from build123d import *

# Parameters (mm, degrees)
SKETCH1_W                   = 36
SKETCH1_H                   = 38
BOSS_EXTRUDE2_DEPTH         = 53
SKETCH3_W                   = 30
SKETCH3_H                   = 35
CUT_EXTRUDE1_DEPTH          = 51
SKETCH4_W                   = 3
SKETCH4_H                   = 30
BOSS_EXTRUDE3_DEPTH         = 33
SKETCH5_W                   = 53
SKETCH5_H                   = 8
CUT_EXTRUDE2_DEPTH          = 52
SKETCH6_W                   = 53
SKETCH6_H                   = 7
BOSS_EXTRUDE4_DEPTH         = 3
CUT_EXTRUDE4_DEPTH          = 79.797208072
CUT_EXTRUDE4_DEPTH_BACK     = 79.797208072
SKETCH8_W                   = 11.5
SKETCH8_H                   = 3
M3_TAPPED_HOLE1_D           = 2.5
M3_TAPPED_HOLE1_DEPTH       = 3
M3_TAPPED_HOLE1_CSINK_D     = 3.05
M3_TAPPED_HOLE1_CSINK_ANGLE = 179
LPATTERN1_COUNT             = 2
LPATTERN1_PITCH             = 24
LPATTERN1_COUNT_DIR2        = 2
LPATTERN1_PITCH_DIR2        = 12
M3_TAPPED_HOLE2_D           = 2.5
M3_TAPPED_HOLE2_DEPTH       = 2
M3_TAPPED_HOLE2_CSINK_D     = 3.05
M3_TAPPED_HOLE2_CSINK_ANGLE = 179
LPATTERN2_COUNT             = 2
LPATTERN2_PITCH             = 16
LPATTERN2_COUNT_DIR2        = 2
LPATTERN2_PITCH_DIR2        = 12
M3_TAPPED_HOLE3_D           = 2.5
M3_TAPPED_HOLE3_CSINK_D     = 3.05
M3_TAPPED_HOLE3_CSINK_ANGLE = 179
LPATTERN3_COUNT             = 2
LPATTERN3_PITCH             = 16
M3_TAPPED_HOLE4_D           = 2.5
M3_TAPPED_HOLE4_CSINK_D     = 3.05
M3_TAPPED_HOLE4_CSINK_ANGLE = 179
LPATTERN4_COUNT             = 2
LPATTERN4_PITCH             = 24
LPATTERN4_COUNT_DIR2        = 2
LPATTERN4_PITCH_DIR2        = 12
SKETCH45_R                  = 1.833333333
CUT_EXTRUDE5_DEPTH          = 74.396185187
LPATTERN5_COUNT             = 2
LPATTERN5_PITCH             = 35
LPATTERN5_COUNT_DIR2        = 2
LPATTERN5_PITCH_DIR2        = 43
CUT_EXTRUDE6_DEPTH          = 75.551995278
CUT_EXTRUDE6_DEPTH_BACK     = 75.551995278
SKETCH46_W                  = 11.5
SKETCH46_H                  = 3.2
CUT_EXTRUDE7_DEPTH          = 74.396185187
CUT_EXTRUDE7_DEPTH_BACK     = 74.396185187
SKETCH47_W                  = 53
SKETCH47_H                  = 7
BOSS_EXTRUDE5_START         = -30
SKETCH49_W                  = 10
SKETCH49_H                  = 36
BOSS_EXTRUDE5_DEPTH         = 3
CUT_EXTRUDE8_DEPTH          = 78.420927403
CUT_EXTRUDE8_DEPTH_BACK     = 78.420927403
SKETCH50_R                  = 1.835


with BuildPart() as part:
    # Sketch1 → Boss-Extrude2 (new body)
    with BuildSketch(Plane(origin=(0, 0, 0), x_dir=(0, 0, -1), z_dir=(1, 0, 0))):
        with Locations((18, 19)):
            Rectangle(SKETCH1_W, SKETCH1_H)
    extrude(amount=BOSS_EXTRUDE2_DEPTH)

    # Sketch3 → Cut-Extrude1 (cut)
    with BuildSketch(Plane(origin=(53, 0, 0), x_dir=(0, 0, -1), z_dir=(1, 0, 0))):
        with Locations((18, 17.5)):
            Rectangle(SKETCH3_W, SKETCH3_H)
    extrude(amount=-CUT_EXTRUDE1_DEPTH, mode=Mode.SUBTRACT)

    # Sketch4 → Boss-Extrude3 (add)
    with BuildSketch(Plane.XY):
        with Locations((51.5, 15)):
            Rectangle(SKETCH4_W, SKETCH4_H)
    extrude(amount=-BOSS_EXTRUDE3_DEPTH)

    # Sketch5 → Cut-Extrude2 (cut)
    with BuildSketch(Plane.XY):
        with Locations((26.5, 34)):
            Rectangle(SKETCH5_W, SKETCH5_H)
    extrude(amount=-CUT_EXTRUDE2_DEPTH, mode=Mode.SUBTRACT)

    # Sketch6 → Boss-Extrude4 (add)
    with BuildSketch(Plane(origin=(0, 0, 0), x_dir=(-1, 0, 0), z_dir=(0, -1, 0))):
        with Locations((-26.5, -3.5)):
            Rectangle(SKETCH6_W, SKETCH6_H)
        with Locations((-26.5, 39.5)):
            Rectangle(SKETCH6_W, SKETCH6_H)
    extrude(amount=-BOSS_EXTRUDE4_DEPTH)

    # Sketch8 → Cut-Extrude4 (cut, two sides: drawn at the far end of the back side and taken through both)
    with BuildSketch(Plane(origin=(0, 0, -43), x_dir=(-1, 0, 0), z_dir=(0, 0, -1)).offset(-CUT_EXTRUDE4_DEPTH_BACK)):
        with Locations((-23.75, 1.5)):
            Rectangle(SKETCH8_W, SKETCH8_H)
    extrude(amount=CUT_EXTRUDE4_DEPTH + CUT_EXTRUDE4_DEPTH_BACK, mode=Mode.SUBTRACT)

    # M3 Tapped Hole1
    with Locations(Plane.XY):
        with Locations((10, 23)):
            m3_tapped_hole1 = CounterSinkHole(M3_TAPPED_HOLE1_D / 2, M3_TAPPED_HOLE1_CSINK_D / 2, depth=M3_TAPPED_HOLE1_DEPTH, counter_sink_angle=M3_TAPPED_HOLE1_CSINK_ANGLE)

    # LPattern1: M3 Tapped Hole1 2 × 2
    with Locations(*[(i * LPATTERN1_PITCH, -j * LPATTERN1_PITCH_DIR2, 0) for i in range(LPATTERN1_COUNT) for j in range(LPATTERN1_COUNT_DIR2) if (i, j) != (0, 0)]):
        add(m3_tapped_hole1, mode=Mode.SUBTRACT)

    # M3 Tapped Hole2
    with Locations(Plane.ZY):
        with Locations((-26, 23)):
            m3_tapped_hole2 = CounterSinkHole(M3_TAPPED_HOLE2_D / 2, M3_TAPPED_HOLE2_CSINK_D / 2, depth=M3_TAPPED_HOLE2_DEPTH, counter_sink_angle=M3_TAPPED_HOLE2_CSINK_ANGLE)

    # LPattern2: M3 Tapped Hole2 2 × 2
    with Locations(*[(0, -j * LPATTERN2_PITCH_DIR2, i * LPATTERN2_PITCH) for i in range(LPATTERN2_COUNT) for j in range(LPATTERN2_COUNT_DIR2) if (i, j) != (0, 0)]):
        add(m3_tapped_hole2, mode=Mode.SUBTRACT)

    # M3 Tapped Hole3 (through all)
    with Locations(Plane(origin=(53, 0, 0), x_dir=(0, 0, -1), z_dir=(1, 0, 0))):
        with Locations((26, 23)):
            m3_tapped_hole3 = CounterSinkHole(M3_TAPPED_HOLE3_D / 2, M3_TAPPED_HOLE3_CSINK_D / 2, counter_sink_angle=M3_TAPPED_HOLE3_CSINK_ANGLE)

    # LPattern3: M3 Tapped Hole3 ×2
    with Locations(*[(0, 0, i * LPATTERN3_PITCH) for i in range(1, LPATTERN3_COUNT)]):
        add(m3_tapped_hole3, mode=Mode.SUBTRACT)

    # M3 Tapped Hole4 (through all)
    with Locations(Plane(origin=(0, 0, -36), x_dir=(-1, 0, 0), z_dir=(0, 0, -1))):
        with Locations((-10, 23)):
            m3_tapped_hole4 = CounterSinkHole(M3_TAPPED_HOLE4_D / 2, M3_TAPPED_HOLE4_CSINK_D / 2, counter_sink_angle=M3_TAPPED_HOLE4_CSINK_ANGLE)

    # LPattern4: M3 Tapped Hole4 2 × 2
    with Locations(*[(i * LPATTERN4_PITCH, -j * LPATTERN4_PITCH_DIR2, 0) for i in range(LPATTERN4_COUNT) for j in range(LPATTERN4_COUNT_DIR2) if (i, j) != (0, 0)]):
        add(m3_tapped_hole4, mode=Mode.SUBTRACT)

    # Sketch45 → Cut-Extrude5 (cut, symmetric)
    with BuildSketch(Plane(origin=(0, 3, 0), x_dir=(1, 0, 0), z_dir=(0, 1, 0))):
        with Locations(Location((8, 39.5, 0), (0, 0, 270))):
            Circle(SKETCH45_R)
    cut_extrude5 = extrude(amount=CUT_EXTRUDE5_DEPTH, both=True, mode=Mode.SUBTRACT)

    # LPattern5: Cut-Extrude5 2 × 2
    with Locations(*[(i * LPATTERN5_PITCH, 0, j * LPATTERN5_PITCH_DIR2) for i in range(LPATTERN5_COUNT) for j in range(LPATTERN5_COUNT_DIR2) if (i, j) != (0, 0)]):
        add(cut_extrude5, mode=Mode.SUBTRACT)

    # Sketch46 → Cut-Extrude6 (cut, two sides: drawn at the far end of the back side and taken through both)
    with BuildSketch(Plane(origin=(0, 0, -36), x_dir=(-1, 0, 0), z_dir=(0, 0, -1)).offset(-CUT_EXTRUDE6_DEPTH_BACK)):
        with Locations((-23.75, 4.6)):
            Rectangle(SKETCH46_W, SKETCH46_H)
    extrude(amount=CUT_EXTRUDE6_DEPTH + CUT_EXTRUDE6_DEPTH_BACK, mode=Mode.SUBTRACT)

    # Sketch47 → Cut-Extrude7 (cut, two sides: drawn at the far end of the back side and taken through both)
    with BuildSketch(Plane(origin=(0, 3, 0), x_dir=(1, 0, 0), z_dir=(0, 1, 0)).offset(-CUT_EXTRUDE7_DEPTH_BACK)):
        with Locations((26.5, 39.5)):
            Rectangle(SKETCH47_W, SKETCH47_H)
        with Locations((26.5, -3.5)):
            Rectangle(SKETCH47_W, SKETCH47_H)
    extrude(amount=CUT_EXTRUDE7_DEPTH + CUT_EXTRUDE7_DEPTH_BACK, mode=Mode.SUBTRACT)

    # Sketch49 → Boss-Extrude5 (add)
    with BuildSketch(Plane(origin=(0, 30, 0), x_dir=(1, 0, 0), z_dir=(0, 1, 0)).offset(BOSS_EXTRUDE5_START)):
        with Locations((-5, 18)):
            Rectangle(SKETCH49_W, SKETCH49_H)
        with Locations((58, 18)):
            Rectangle(SKETCH49_W, SKETCH49_H)
    extrude(amount=BOSS_EXTRUDE5_DEPTH)

    # Sketch50 → Cut-Extrude8 (cut, two sides: drawn at the far end of the back side and taken through both)
    with BuildSketch(Plane(origin=(0, 3, 0), x_dir=(1, 0, 0), z_dir=(0, 1, 0)).offset(-CUT_EXTRUDE8_DEPTH_BACK)):
        with Locations(Location((-5, 28, 0), (0, 0, 270))):
            Circle(SKETCH50_R)
        with Locations(Location((-5, 8, 0), (0, 0, 270))):
            Circle(SKETCH50_R)
        with Locations(Location((58, 8, 0), (0, 0, 270))):
            Circle(SKETCH50_R)
        with Locations(Location((58, 28, 0), (0, 0, 270))):
            Circle(SKETCH50_R)
    extrude(amount=CUT_EXTRUDE8_DEPTH + CUT_EXTRUDE8_DEPTH_BACK, mode=Mode.SUBTRACT)


solid = part.part
The listing builds one solid part. Answer for the finished solid, in the listing's coordinates (mm). A direction names the side the tool comes from. Round coordinates to 2 decimals unless told otherwise and drop trailing zeros. Write each loop counter-clockwise with the first axis right and the second up, starting at its lowest first coordinate (ties: lowest second). Pieces come first, ordered by that corner, then holes. Notation, with made-up numbers: (22.5, 77.5) - (46.5, 77.5) arc R24 cw to (46.5, 102.5) - close; hole circle Ø2 at (30, 64.5). An arc over 180 degrees is marked (long way). Use one line per item in the form item = value. Start each with the question number.
Item 1: Flat-ended cylindrical pins translate along their axes: pin 1 Ø2 at (y, z) = (25, -12) entering from -X; pin 2 Ø3.5 at (x, z) = (25.5, -35) entering from -Y; pin 3 Ø3 at (y, z) = (11, -26) entering from +X. Find the tip coordinate at first contact, or state that the pin passes through.
Item 2: Find the intervals of material crossed by line 1 (Y direction, x = 34, z = -1); line 2 (X direction, y = 23, z = -35.4); line 3 (Z direction, x = 0.85, y = 11), in increasing order. Write a range as [from, to].
Item 3: Determine the mould class of faces 1 (the flat face through (-5, 3, -18)), 2 (the flat face through (26, 15, -36)), 3 (the cylindrical face through (57.297, 1.479, -26.305)) for opening direction Z: +Z half, -Z half, draft (parallel to the pull), parting line (faces both ways), or undercut.
Item 4: A cutting plane is placed at A-A (x = -5). Write down the section's boundary in (y, z) (3 decimals), plus the area to 3 significant figures.
Item 5: A tool of negligible diameter and unlimited length cuts with its end or side. For faces 4 (the cylindrical face through (34.672, 12.054, -34.478)), 5 (the flat face through (29.5, 3, -1)), 6 (the flat face through (53, 16, -18)), from which of +Z, -Z, +X, -X, +Y, -Y can it reach the whole face along a straight path? Write none if from no direction.
Item 6: A cutting plane is placed at D-D (x = 10). Give the number of separate pieces and of enclosed holes in the cut face, plus the area to 3 significant figures.
Item 7: A cutting plane is placed at C-C (z = -19.5). Write down the section's boundary in (x, y).
Item 8: A cutting plane is placed at B-B (y = 17.5). Write down the section's boundary in (x, z), plus the area to 3 significant figures.
The answers:
q1.pin_1 = 0
q1.pin_2 = 6.2
q1.pin_3 = 53
q2.line_1 = [0, 9.75], [12.25, 21.75], [24.25, 30]
q2.line_2 = [0, 8.75], [11.25, 32.75], [35.25, 53]
q2.line_3 = [-36, -27.25], [-24.75, -11.25], [-8.75, 0]
q3.face_1 = draft
q3.face_2 = -Z half
q3.face_3 = undercut
q4.outline = (0, -36) - (3, -36) - (3, -29.835) - (0, -29.835) - close; (0, -26.165) - (3, -26.165) - (3, -9.835) - (0, -9.835) - close; (0, -6.165) - (3, -6.165) - (3, 0) - (0, 0) - close
q4.area = 86.0 mm^2
q5.face_4 = +Z, -Z
q5.face_5 = +Z, -Z, -Y
q5.face_6 = +Z, -Z, +X, +Y
q6.separate_pieces = 6
q6.enclosed_holes = 0
q6.area = 150 mm^2
q7.outline = (-10, 0) - (2, 0) - (2, 30) - (0, 30) - (0, 3) - (-10, 3) - close; (50, 0) - (63, 0) - (63, 3) - (53, 3) - (53, 30) - (50, 30) - close
q8.outline = (0, -36) - (53, -36) - (53, 0) - (0, 0) - close; hole (2, -33) - (50, -33) - (50, -3) - (2, -3) - close
q8.area = 468 mm^2
